Autodesk Inventor part; units mm, degrees
ref_plane "YZ Plane" through (0, 0, 0) normal (1, 0, 0) x (0, 1, 0)
ref_plane "XZ Plane" through (0, 0, 0) normal (0, 1, 0) x (-1, 0, 0)
ref_plane "XY Plane" through (0, 0, 0) normal (0, 0, 1) x (1, 0, 0)
sketch "Sketch1" plane through (0, 0, 0) normal (0, 1, 0) x (-1, 0, 0)
  circle A0 centre (59.7558, 0) radius 1.6
  circle A1 centre (0, 0) radius 1.6
  arc A2 (59.7558, -5) -> (59.7558, 5) centre (59.7558, 0) ccw
  arc A3 (0, 5) -> (0, -5) centre (0, 0) ccw
  line L0 (59.7558, 5) -> (0, 5)
  line L1 (59.7558, -5) -> (0, -5)
  dimension "d0" = 3.2
  dimension "d1" = 3.2
  dimension "d2" = 59.7557
  dimension "d12" = 10
  dimension "d13" = 10
extrude "Extrusion1" add sketch "Sketch1" along normal blind 3.2
equation "\"d13\" = d12"
properties part number "portabateria"
CAD build for the part. Positions are in the model's coordinates, mm. Give positions to 0.01 mm unless a question says otherwise; leave off trailing zeros. Write each loop counter-clockwise with the first axis right and the second up, starting at its lowest first coordinate (ties: lowest second). Pieces come first, ordered by that corner, then holes. Notation, with made-up numbers: (50.25, 57) -> (92.25, 57) arc R23 ccw to (92.25, 66) -> close; hole circle Ø8 at (86.5, 48.5). An arc over 180 degrees is marked (long way). Return JSON: item names as keys, results as strings.
Item 1: Two-plate mould, pull along X, no slides. Class faces 1 (the cylindrical face through (-64.755, 1.578, 0.11)), 2 (the flat face through (-30, 2, -5)), 3 (the cylindrical face through (1.27, 1.58, 0.97)): +X half, -X half, draft (parallel to the pull), parting line (faces both ways), or undercut.
Answer below:
{"face 1": "-X half", "face 2": "draft", "face 3": "undercut"}
Item 2: Band-saw the part on A-A (z = 0). List the corners of the cut face in (x, y).
Answer below:
{"outline": "(-64.76, 0) -> (-61.36, 0) -> (-61.36, 3.2) -> (-64.76, 3.2) -> close; (-58.16, 0) -> (-1.6, 0) -> (-1.6, 3.2) -> (-58.16, 3.2) -> close; (1.6, 0) -> (5, 0) -> (5, 3.2) -> (1.6, 3.2) -> close"}
Item 3: Band-saw the part on B-B (y = 2.5). List the corners of the cut face in (x, z), then the cut area to 3 significant figures.
Answer below:
{"outline": "(-59.76, -5) -> (0, -5) arc R5 ccw to (0, 5) -> (-59.76, 5) arc R5 ccw to start; hole circle Ø3.2 at (-59.76, 0); hole circle Ø3.2 at (0, 0)", "area": "660 mm2"}
Item 4: Drill centre lines: probe 1 along Z at (x, y) = (0, 1.15); probe 2 along X at (y, z) = (1.9, 0.5); probe 3 along X at (y, z) = (0.7, 0.25). Where is each one in solid material? Low to high.
Answer below:
{"probe 1": "z = -5 to -1.6, 1.6 to 5", "probe 2": "x = -64.73 to -61.28, -58.24 to -1.52, 1.52 to 4.97", "probe 3": "x = -64.75 to -61.34, -58.18 to -1.58, 1.58 to 4.99"}
Item 5: Band-saw the part on C-C (z = 4). List the corners of the cut face in (x, y).
Answer below:
{"outline": "(-62.76, 0) -> (3, 0) -> (3, 3.2) -> (-62.76, 3.2) -> close"}
